```python
from build123d import *

# Parameters (mm, degrees)
F0_W     = 97.5
F0_H     = 50
F1_DEPTH = 10
F2_T     = -5
F3_W     = 5
F3_H     = 5
F4_DEPTH = 5
F6_D     = 5
F7_R     = 10


with BuildPart() as f1:
    # F0 (on Top) → F1 (new body)
    with BuildSketch(Plane.XY):
        with Locations((48.75, 25)):
            Rectangle(F0_W, F0_H)
    extrude(amount=F1_DEPTH)

    # F2
    f2_openings = [f1.faces().sort_by_distance(p)[0] for p in [
        (97.5, 25, 5),
        (48.75, 50, 5),
        (48.75, 25, 10),
    ]]
    offset(amount=F2_T, openings=f2_openings)

    # F3 (on face) → F4 (cut)
    with BuildSketch(Plane.XY.offset(10)):
        with Locations((6, 6)):
            Rectangle(F3_W, F3_H)
    extrude(amount=-F4_DEPTH, mode=Mode.SUBTRACT)

    # F6 (through all)
    with Locations(Plane.XY.offset(5)):
        with Locations((57, 42.5), (89, 42.5)):
            Hole(F6_D / 2)

    # F7
    f7_edges = [f1.edges().sort_by_distance(p)[0] for p in [
        (97.5, 50, 2.5),
    ]]
    fillet(f7_edges, radius=F7_R)


solid = f1.part
```
Model file for the job. Use its own axes, mm. A direction names the side the tool comes from. Round coordinates to 2 decimals unless told otherwise and drop trailing zeros. Loops run counter-clockwise (first coordinate to the right, second up) from the corner with the lowest first, then second, coordinate; pieces in that order, holes last. Notation, with made-up numbers: M -39.75,-13 L -11.75,-13 A22 cw -11.75,16 Z; hole C 38.5,15.25 d4. An arc over 180 degrees is marked long. Put each result on its own line as item: value. Start each with the question number.
Item 1: 3-axis set-ups, long thin cutter, end or side, ignore diameter. For faces 1 (the face through (97.5, 20, 3)), 2 (the face through (6, 3.5, 8)), 3 (the face through (5, 29, 7)): which of +Z, -Z, +X, -X, +Y, -Y reach the whole face in a straight line?
Item 2: Cut at A-A (x = 57). List the corners of the cut face in (y, z), then the cut area to 3 significant figures.
Item 3: Drop flat-ended pins along their axis: P1, Ø12, axis at x = 34, y = 20.5, coming from the +Z side; P2, Ø1.5, axis at y = 6, z = 8.5, coming from the +X side; P3, Ø1.5, axis at y = 28, z = 7.5, coming from the +X side. Give the stop position or say it passes through.
Item 4: Cut at B-B (y = 44). List the corners of the cut face in (x, z).
Item 5: Cut at D-D (y = 23.5). List the corners of the cut face in (x, z), then the cut area to 4 significant figures.
Item 6: Drill centre lines: line 1 along Y through (x, z) = (57, 2.15); line 2 along X through (y, z) = (27, 7.75); line 3 along Y through (x, z) = (6.5, 7.75). Where is each one in solid material? Low to high.
Item 7: Mould opens along Y. For faces 4 (the face through (3.5, 6, 8)), 5 (the face through (52, 5, 7)), 6 (the face through (48, 25, 0)) say: released by +Y, released by -Y, zero draft, split by the parting line, or undercut.
Item 8: Cut at C-C (z = 8.75). List the corners of the cut face in (x, y), then the cut area to 3 significant figures.
Answer block:
1. face 1: +Z, -Z, +X, +Y, -Y
1. face 2: +Z
1. face 3: +Z, +X, +Y
2. outline: M 0,0 L 40,0 L 40,5 L 5,5 L 5,10 L 0,10 Z; M 45,0 L 50,0 L 50,5 L 45,5 Z
2. area: 250 mm2
3. P1: z = 5
3. P2: x = 3.5
3. P3: x = 5
4. outline: M 0,0 L 55,0 L 55,5 L 5,5 L 5,10 L 0,10 Z; M 59,0 L 87,0 L 87,5 L 59,5 Z; M 91,0 L 96.67,0 L 96.67,5 L 91,5 Z
5. outline: M 0,0 L 97.5,0 L 97.5,5 L 5,5 L 5,10 L 0,10 Z
5. area: 512.5 mm2
6. line 1: 0 to 40, 45 to 50
6. line 2: 0 to 5
6. line 3: 0 to 3.5
7. face 4: undercut
7. face 5: released by +Y
7. face 6: zero draft
8. outline: M 0,0 L 97.5,0 L 97.5,5 L 8.5,5 L 8.5,3.5 L 3.5,3.5 L 3.5,8.5 L 5,8.5 L 5,50 L 0,50 Z
8. area: 700 mm2
